Input: part model. Units: mm. Frame: model coordinates. A direction names the side the tool comes from. Coordinates: 2 decimals unless noted, no trailing zeros. Loops run counter-clockwise (first coordinate to the right, second up) from the corner with the lowest first, then second, coordinate; pieces in that order, holes last.
Item 1: Contact query for flat-ended pins moving along their axis: P1, Ø1.6, axis at y = 23.5, z = -7.5, coming from the +X side; P2, Ø1, axis at x = -4, y = 24.5, coming from the +Z side; P3, Ø5, axis at y = 32, z = -5.5, coming from the -X side. Output: stop coordinate, or through.
Item 2: Pull-direction query (X, two-part tool) for faces 1 (the flat face through (2.5, 21, -8)), 2 (the flat face through (0, 21, -6.538)), 3 (the flat face through (0, 41, 0)), 4 (the conical face through (0.336, 40.681, 8.313)); classes: released by +X, released by -X, zero draft, split by the parting line, or undercut.
Item 3: Section B-B on y = 35. Return loops of the section in (x, z), and give its area (3 significant figures).
Item 4: Reachability of faces 5 (the flat face through (-2.5, 21, -8)), 6 (the flat face through (0, 0, 0)) from +Z, -Z, +X, -X, +Y, -Y: full face, straight path, thin tool, end or side. Return the list, or none.
Item 5: Ray query, line 1 along X through (y, z) = (8.5, 0.25); line 2 along Z through (x, y) = (5.5, 19); line 3 along X through (y, z) = (34.5, 3.75). Return the intervals inside material, ascending.
Item 6: Section A-A on x = 0. Return loops of the section in (y, z).
```python
from build123d import *

# Parameters (mm, degrees)
SKETCH_1_R          = 10
EXTRUDE_1_DEPTH     = 41
SKETCH_2_W          = 5
SKETCH_2_H          = 3.914156893
CUT_EXTRUDE_1_DEPTH = 48
CHAMFER_1_SIZE      = 2


with BuildPart() as part:
    # Эскиз1 → Бобышка-Вытянуть1 (new body)
    with BuildSketch(Plane(origin=(0, 0, 0), x_dir=(1, 0, 0), z_dir=(0, 1, 0))):
        with Locations(Location((0, 0, 0), (0, 0, 270))):
            Circle(SKETCH_1_R)
    extrude(amount=EXTRUDE_1_DEPTH)

    # Эскиз2 → Вырез-Вытянуть1 (cut)
    with BuildSketch(Plane(origin=(0, 41, 0), x_dir=(1, 0, 0), z_dir=(0, 1, 0))):
        with Locations((0, 8.495426862)):
            Rectangle(SKETCH_2_W, SKETCH_2_H)
    extrude(amount=-CUT_EXTRUDE_1_DEPTH, mode=Mode.SUBTRACT)

    # Фаска1
    chamfer_1_edges = [part.edges().sort_by_distance(p)[0] for p in [
        (0, 41, 10),
    ]]
    chamfer(chamfer_1_edges, length=CHAMFER_1_SIZE)


solid = part.part
```
Results found:
1. P1: stops at x = 7.42
1. P2: stops at z = 9.37
1. P3: stops at x = -9.54
2. face 1: undercut
2. face 2: undercut
2. face 3: zero draft
2. face 4: split by the parting line
3. outline: (-2.5, -9.68) - (-2.5, -6.54) - (2.5, -6.54) - (2.5, -9.68) arc R10 ccw (long way) to start
3. area: 297 mm2
4. face 5: -Z, +Y, -Y
4. face 6: +Z, -Z, +X, -X, -Y
5. line 1: x = -10 to 10
5. line 2: z = -8.35 to 8.35
5. line 3: x = -9.27 to 9.27
6. outline: (0, -6.54) - (41, -6.54) - (41, 8) - (39, 10) - (0, 10) - close
